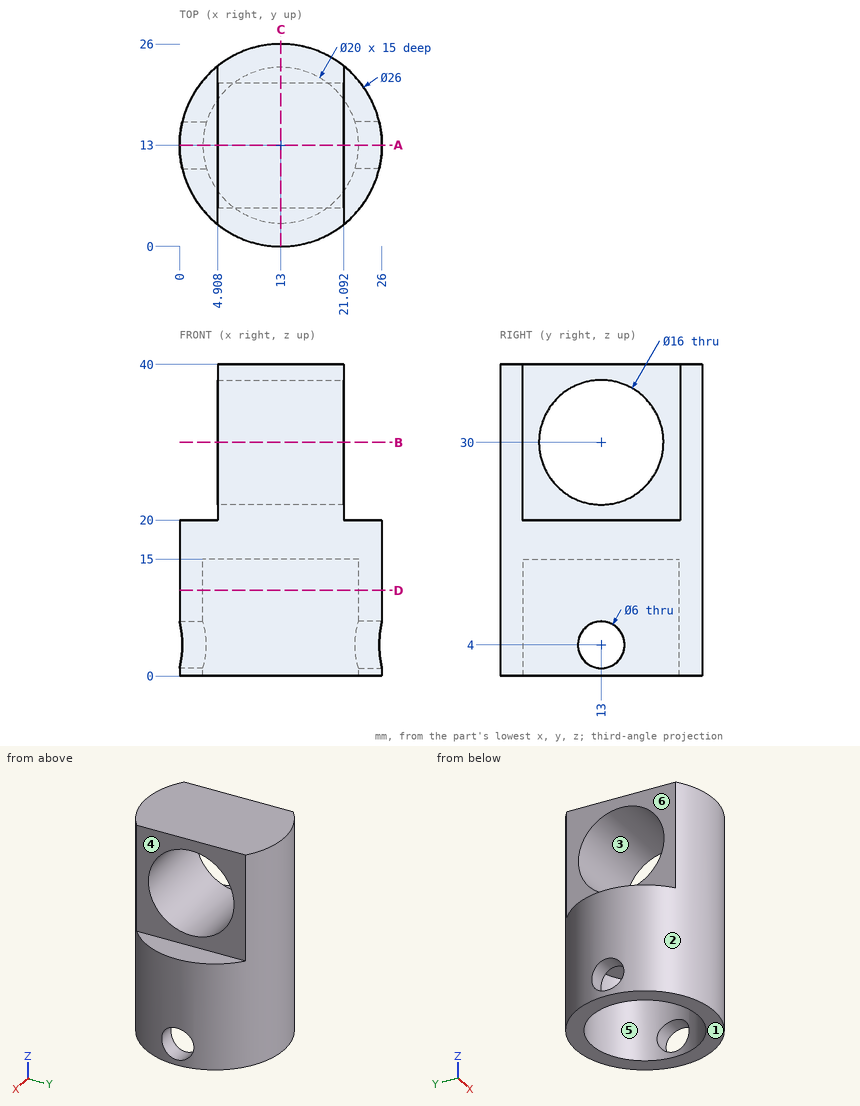
Print and shaded views of the part. All mm, measured from the part's lowest x, y and z. A direction names the side the tool comes from. Coordinates: 2 decimals unless noted, no trailing zeros. Order: outer loops, then holes, each group sorted by start corner. A loop starts at its lowest first (then second) coordinate and runs counter-clockwise, first axis right, second up. Notation, with made-up numbers: (69.25, -29.75) - (120.25, -29.75) arc R37 ccw to (120.25, 7.25) - close; hole circle Ø8 at (11, -38.5). An arc over 180 degrees is marked (long way). Put each result on its own line as item: value.
1. Saw through at C-C (x = 13). Write the cut outline in (y, z), and give its area (3 significant figures).
Answer sheet:
outline: (0, 0) - (3, 0) - (3, 15) - (23, 15) - (23, 0) - (26, 0) - (26, 40) - (0, 40) - close; hole circle Ø16 at (13, 30)
area: 539 mm^2
2. Saw through at A-A (y = 13). Write the cut outline in (x, z).
Answer sheet:
outline: (0, 0) - (3, 0) - (3, 1) - (0, 1) - close; (0, 7) - (3, 7) - (3, 15) - (23, 15) - (23, 7) - (26, 7) - (26, 20) - (21.09, 20) - (21.09, 22) - (4.91, 22) - (4.91, 20) - (0, 20) - close; (4.91, 38) - (21.09, 38) - (21.09, 40) - (4.91, 40) - close; (23, 0) - (26, 0) - (26, 1) - (23, 1) - close
3. Saw through at B-B (z = 30). Write the cut outline in (x, y) (1 decimal).
Answer sheet:
outline: (4.9, 2.8) arc R13 ccw to (21.1, 2.8) - (21.1, 5) - (4.9, 5) - close; (4.9, 21) - (21.1, 21) - (21.1, 23.2) arc R13 ccw to (4.9, 23.2) - close
4. Saw through at D-D (z = 11). Write the cut outline in (x, y).
Answer sheet:
outline: circle Ø26 at (13, 13); hole circle Ø20 at (13, 13)
5. Probe line 1 along X through (y, z) = (13, 7.5); line 2 along X through (y, z) = (6.25, 38.5); line 3 along X through (y, z) = (7.5, 11). List the from-to ranges inside material, lowest first. Write a range as [from, to].
Answer sheet:
line 1: x = [0, 3], [23, 26]
line 2: x = [4.91, 21.09]
line 3: x = [1.22, 4.65], [21.35, 24.78]
6. Drop flat-ended pins along their axis: P1, Ø5, axis at y = 2.5, z = 7, coming from the -X side; P2, Ø5.5, axis at x = 2, y = 18, coming from the +Z side; P3, Ø12, axis at x = 21, z = 21, coming from the -Y side (1 decimal). Give the stop position or say it passes through.
Answer sheet:
P1: stops at x = 2.75
P2: stops at z = 20
P3: stops at y = 0.2
7. Tool access for the marked faces 4, 5 and 6: list every direction of +Z, -Z, +X, -X, +Y, -Y with a clear straight run to the whole face (end or side of a thin tool).
Answer sheet:
face 4: +Z, +X, +Y, -Y
face 5: -Z
face 6: +Z, -X, +Y, -Y
8. Pull direction Y, two halves, no side cores. Call the marked faces 1, 2 and 3: pulls with the +Y half, pulls with the -Y half, needs draft (parallel to the pull), parting line crosses it, or undercut.
Answer sheet:
face 1: needs draft
face 2: parting line crosses it
face 3: undercut
